```python
from build123d import *

# Parameters (mm, degrees)
SZKIC1_W                    = 596
SZKIC1_H                    = 396
DODANIE_WYCI_GNI_CIE1_DEPTH = 46
SZKIC2_R                    = 21
WYTNIJ_WYCI_GNI_CIE1_DEPTH  = 46
SZKIC3_R                    = 21
WYTNIJ_WYCI_GNI_CIE2_DEPTH  = 46
SZKIC4_R                    = 21
WYTNIJ_WYCI_GNI_CIE3_DEPTH  = 46
SZKIC5_R                    = 21
WYTNIJ_WYCI_GNI_CIE4_DEPTH  = 46
SZKIC6_W                    = 46
SZKIC6_H                    = 9
SZKIC7_W                    = 46
SZKIC7_H                    = 9
SZKIC8_W                    = 46
SZKIC8_H                    = 9
SZKIC9_W                    = 46
SZKIC9_H                    = 9


with BuildPart() as part:
    # Szkic1 → Dodanie-wyci_gni_cie1 (new body)
    with BuildSketch(Plane.XY):
        Rectangle(SZKIC1_W, SZKIC1_H)
    extrude(amount=DODANIE_WYCI_GNI_CIE1_DEPTH)

    # Szkic2 → Wytnij-wyci_gni_cie1 (cut)
    with BuildSketch(Plane.XY.offset(46)):
        with Locations((262, 162)):
            Circle(SZKIC2_R)
    extrude(amount=-WYTNIJ_WYCI_GNI_CIE1_DEPTH, mode=Mode.SUBTRACT)

    # Szkic3 → Wytnij-wyci_gni_cie2 (cut)
    with BuildSketch(Plane.XY.offset(46)):
        with Locations((262, -162)):
            Circle(SZKIC3_R)
    extrude(amount=-WYTNIJ_WYCI_GNI_CIE2_DEPTH, mode=Mode.SUBTRACT)

    # Szkic4 → Wytnij-wyci_gni_cie3 (cut)
    with BuildSketch(Plane.XY.offset(46)):
        with Locations((-262, -162)):
            Circle(SZKIC4_R)
    extrude(amount=-WYTNIJ_WYCI_GNI_CIE3_DEPTH, mode=Mode.SUBTRACT)

    # Szkic5 → Wytnij-wyci_gni_cie4 (cut)
    with BuildSketch(Plane.XY.offset(46)):
        with Locations((-262, 162)):
            Circle(SZKIC5_R)
    extrude(amount=-WYTNIJ_WYCI_GNI_CIE4_DEPTH, mode=Mode.SUBTRACT)

    # Szkic6 → Wyci_cie-obr_t1 (revolve, cut)
    with BuildSketch(Plane(origin=(215, 0, 0), x_dir=(0, 0, -1), z_dir=(1, 0, 0)), mode=Mode.PRIVATE) as wyci_cie_obr_t1_sk:
        with Locations((-23, 166.5)):
            Rectangle(SZKIC6_W, SZKIC6_H)
    revolve(wyci_cie_obr_t1_sk.sketch.rotate(Axis((215, 162, 0), (0, 0, 1)), 270), axis=Axis((215, 162, 0), (0, 0, 1)), mode=Mode.SUBTRACT)

    # Szkic7 → Wyci_cie-obr_t2 (revolve, cut)
    with BuildSketch(Plane(origin=(215, 0, 0), x_dir=(0, 0, -1), z_dir=(1, 0, 0)), mode=Mode.PRIVATE) as wyci_cie_obr_t2_sk:
        with Locations((-23, -166.5)):
            Rectangle(SZKIC7_W, SZKIC7_H)
    revolve(wyci_cie_obr_t2_sk.sketch.rotate(Axis((215, -162, 46), (0, 0, -1)), 90), axis=Axis((215, -162, 46), (0, 0, -1)), mode=Mode.SUBTRACT)

    # Szkic8 → Wyci_cie-obr_t3 (revolve, cut)
    with BuildSketch(Plane(origin=(-215, 0, 0), x_dir=(0, 0, -1), z_dir=(1, 0, 0)), mode=Mode.PRIVATE) as wyci_cie_obr_t3_sk:
        with Locations((-23, 166.5)):
            Rectangle(SZKIC8_W, SZKIC8_H)
    revolve(wyci_cie_obr_t3_sk.sketch.rotate(Axis((-215, 162, 0), (0, 0, 1)), 270), axis=Axis((-215, 162, 0), (0, 0, 1)), mode=Mode.SUBTRACT)

    # Szkic9 → Wyci_cie-obr_t4 (revolve, cut)
    with BuildSketch(Plane(origin=(-215, 0, 0), x_dir=(0, 0, -1), z_dir=(1, 0, 0)), mode=Mode.PRIVATE) as wyci_cie_obr_t4_sk:
        with Locations((-23, -166.5)):
            Rectangle(SZKIC9_W, SZKIC9_H)
    revolve(wyci_cie_obr_t4_sk.sketch.rotate(Axis((-215, -162, 46), (0, 0, -1)), 90), axis=Axis((-215, -162, 46), (0, 0, -1)), mode=Mode.SUBTRACT)


solid = part.part
```
Build history of the part. All positions in model axes, mm. Round coordinates to 2 decimals unless told otherwise and drop trailing zeros. Loops run counter-clockwise (first coordinate to the right, second up) from the corner with the lowest first, then second, coordinate; pieces in that order, holes last.
Item 1: Saw through at C-C (y = -162). List the corners of the cut face in (x, z), then the cut area to 3 significant figures.
Item 2: Drill centre lines: line 1 along Y through (x, z) = (-262, 28); line 2 along X through (y, z) = (-177.5, 9.5); line 3 along Y through (x, z) = (213, 37.5). Where is each one in solid material? Low to high.
Item 3: Pin check, flat tip, straight feed: P1, Ø11, axis at x = -215, y = 162, coming from the +Z side. Stop position of the tip, or through.
Item 4: Saw through at A-A (x = -262). List the corners of the cut face in (y, z), then the cut area to 3 significant figures.
Item 5: Two-plate mould, pull along X, no slides. Class faces 1 (the face through (-4, -198, 23)), 2 (the face through (-277.48, 176.19, 23.32)), 3 (the face through (298, -3, 23)): released by +X, released by -X, zero draft, split by the parting line, or undercut.
Item 6: Saw through at D-D (x = 215). List the corners of the cut face in (y, z).
Item 7: Saw through at B-B (z = 17). State how many separate pieces and enclosed holes the cut face has, then the cut area to 3 significant figures.
Worked answers:
1. outline: (-298, 0) - (-283, 0) - (-283, 46) - (-298, 46) - close; (-241, 0) - (-224, 0) - (-224, 46) - (-241, 46) - close; (-206, 0) - (206, 0) - (206, 46) - (-206, 46) - close; (224, 0) - (241, 0) - (241, 46) - (224, 46) - close; (283, 0) - (298, 0) - (298, 46) - (283, 46) - close
1. area: 21,900 mm2
2. line 1: y = -198 to -183, -141 to 141, 183 to 198
2. line 2: x = -298 to -276.17, -247.83 to 247.83, 276.17 to 298
2. line 3: y = -198 to -170.77, -153.23 to 153.23, 170.77 to 198
3. P1: passes through
4. outline: (-198, 0) - (-183, 0) - (-183, 46) - (-198, 46) - close; (-141, 0) - (141, 0) - (141, 46) - (-141, 46) - close; (183, 0) - (198, 0) - (198, 46) - (183, 46) - close
4. area: 14,400 mm2
5. face 1: zero draft
5. face 2: undercut
5. face 3: released by +X
6. outline: (-198, 0) - (-171, 0) - (-171, 46) - (-198, 46) - close; (-153, 0) - (153, 0) - (153, 46) - (-153, 46) - close; (171, 0) - (198, 0) - (198, 46) - (171, 46) - close
7. separate pieces: 1
7. enclosed holes: 8
7. area: 229,000 mm2
